```python
from build123d import *

# Parameters (mm, degrees)
F0_R          = 25.91
F1_DEPTH      = 7
F1_DEPTH_BACK = 7
F2_R          = 17
F3_DEPTH      = 7
F3_DEPTH_BACK = 7
F6_START      = -6
F5_W          = 8
F5_H          = 14
F6_DEPTH      = 14
F7_R          = 2.15
F8_DEPTH      = 30
F8_DEPTH_BACK = 30
F9_W          = 10
F9_H          = 14
F10_DEPTH     = 10
F11_W         = 75.513869524
F11_H         = 46.2215282023
F12_DEPTH     = 30


with BuildPart() as f1:
    # F0 (on Front) → F1 (new body, two sides)
    with BuildSketch(Plane.XZ) as f1_sk:
        Circle(F0_R)
    extrude(amount=F1_DEPTH)
    extrude(f1_sk.sketch, amount=-F1_DEPTH_BACK)

    # F2 (on Front) → F3 (cut, two sides)
    with BuildSketch(Plane.XZ) as f3_sk:
        Circle(F2_R)
    extrude(amount=-F3_DEPTH, mode=Mode.SUBTRACT)
    extrude(f3_sk.sketch, amount=F3_DEPTH_BACK, mode=Mode.SUBTRACT)

    # F5 (on face) → F6 (join)
    with BuildSketch(Plane.XY.offset(F6_START)):
        with Locations((-19.91, 0)):
            Rectangle(F5_W, F5_H)
        with Locations((19.91, 0)):
            Rectangle(F5_W, F5_H)
    extrude(amount=-F6_DEPTH)

    # F7 (on face) → F8 (cut, two sides)
    with BuildSketch(Plane.XY) as f8_sk:
        with Locations((-19.1982129737, 0)):
            Circle(F7_R)
        with Locations((19.0490627756, 0)):
            Circle(F7_R)
    extrude(amount=F8_DEPTH, mode=Mode.SUBTRACT)
    extrude(f8_sk.sketch, amount=-F8_DEPTH_BACK, mode=Mode.SUBTRACT)

    # F9 (on face) → F10 (cut)
    with BuildSketch(Plane(origin=(0, 0, -20), x_dir=(1, 0, 0), z_dir=(0, 0, -1))):
        with Locations((-18.91, 0)):
            Rectangle(F9_W, F9_H)
        with Locations((18.91, 0)):
            Rectangle(F9_W, F9_H)
    extrude(amount=F10_DEPTH, mode=Mode.SUBTRACT)

    # F11 (on face) → F12 (cut)
    with BuildSketch(Plane.XY):
        Rectangle(F11_W, F11_H)
    extrude(amount=F12_DEPTH, mode=Mode.SUBTRACT)


solid = f1.part
```
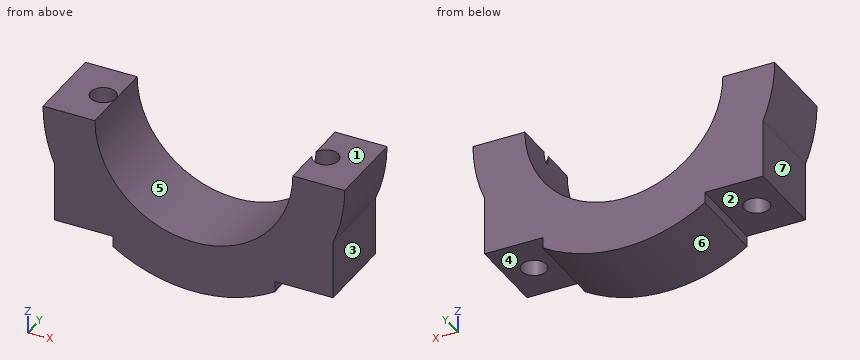
Model file for the job. Use its own axes, mm. Face numbers are marked on the shaded views. A direction names the side the tool comes from. Give positions to 0.01 mm unless a question says otherwise; leave off trailing zeros. Order: outer loops, then holes, each group sorted by start corner. A loop starts at its lowest first (then second) coordinate and runs counter-clockwise, first axis right, second up.
1) Saw through at A-A, the plane z = -6. Write the cut outline in (x, y).
2) Saw through at D-D, the plane y = 4. Write the cut outline in (x, z), then the cut area to 3 significant figures.
3) Pin check, flat tips, straight feed: pin 1 (6 mm diameter, centred on x = 1, z = -12, fed in from +Y); pin 2 (5 mm diameter, centred on y = -0.5, z = -17, fed in from -X); pin 3 (6 mm diameter, centred on y = -4, z = -7.5, fed in from -X); pin 4 (0.9 mm diameter, centred on y = -2, z = -20.5, fed in from +X). Stop position of each tip, or through.
4) Mould opens along X. For the marked faces 4, 5, 6 and 7 say: +X half, -X half, draft (parallel to the pull), parting line (faces both ways), or undercut.
5) Saw through at B-B, the plane x = -19. Write the cut outline in (y, z), then the cut area to 3 significant figures.
6) Wall check: probe 1 along X at (y, z) = (-1.5, -9.5); probe 2 along X at (y, z) = (1.5, -6); probe 3 along X at (y, z) = (-5, -1.75). Give the ranges that are in metal, low to high.
7) 3-axis set-ups, long thin cutter, end or side, ignore diameter. For the marked faces 1, 2 and 3: which of +Z, -Z, +X, -X, +Y, -Y reach the whole face in a straight line?
8) Saw through at C-C, the plane y = -1.5. Write the cut outline in (x, z), then the cut area to 3 significant figures.
Computed:
1. outline: (-25.21, -7) - (-15.91, -7) - (-15.91, 7) - (-25.21, 7) - close; (15.91, -7) - (25.21, -7) - (25.21, 7) - (15.91, 7) - close; hole circle Ø4.3 at (-19.2, 0); hole circle Ø4.3 at (19.05, 0)
2. outline: (-25.91, 0) arc R25.91 ccw to (-23.91, -9.98) - (-23.91, -20) - (-13.91, -20) - (-13.91, -21.86) arc R25.91 ccw to (13.91, -21.86) - (13.91, -20) - (23.91, -20) - (23.91, -9.98) arc R25.91 ccw to (25.91, 0) - (17, 0) arc R17 cw to (-17, 0) - close
2. area: 657 mm2
3. pin 1: passes through
3. pin 2: stops at x = -23.91
3. pin 3: stops at x = -25.52
3. pin 4: stops at x = 13.91
4. face 4: draft
4. face 5: undercut
4. face 6: parting line
4. face 7: -X half
5. outline: (-7, -20) - (-2.14, -20) - (-2.14, 0) - (-7, 0) - close; (2.14, -20) - (7, -20) - (7, 0) - (2.14, 0) - close
5. area: 194 mm2
6. probe 1: x = -24.11 to -20.74, -17.66 to -14.1, 14.1 to 17.51, 20.59 to 24.11
6. probe 2: x = -25.21 to -20.74, -17.66 to -15.91, 15.91 to 17.51, 20.59 to 25.21
6. probe 3: x = -25.85 to -16.91, 16.91 to 25.85
7. face 1: +Z, +X, -X, +Y, -Y
7. face 2: -Z, -X, +Y, -Y
7. face 3: -Z, +X, +Y, -Y
8. outline: (-25.91, 0) arc R25.91 ccw to (-23.91, -9.98) - (-23.91, -20) - (-20.74, -20) - (-20.74, 0) - close; (-17.66, -20) - (-13.91, -20) - (-13.91, -21.86) arc R25.91 ccw to (13.91, -21.86) - (13.91, -20) - (17.51, -20) - (17.51, 0) - (17, 0) arc R17 cw to (-17, 0) - (-17.66, 0) - close; (20.59, -20) - (23.91, -20) - (23.91, -9.98) arc R25.91 ccw to (25.91, 0) - (20.59, 0) - close
8. area: 534 mm2
